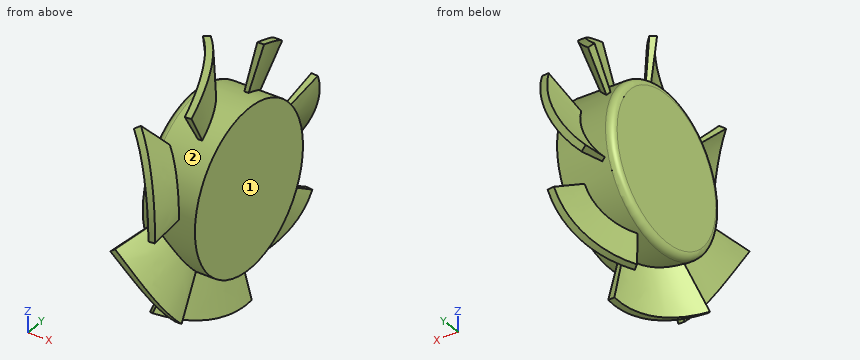
from build123d import *

# Parameters (mm, degrees)
SKETCH5_W                  = 8
SKETCH5_H                  = 11.5
CIRPATTERN1_COUNT          = 7
SKETCH_CUT_BLADE_OUTSIDE_W = 50.999
SKETCH_CUT_BLADE_OUTSIDE_H = 50.116
SKETCH_CUT_BLADE_OUTSIDE_R = 18
CUT_FAN_BLADE_DEPTH        = 30.009117079
COSMETIC_FILLET_R          = 1


with BuildPart() as part:
    # Sketch5 → Body (revolve)
    with BuildSketch(Plane.XY, mode=Mode.PRIVATE) as body_sk:
        with Locations((-6, 5.75)):
            Rectangle(SKETCH5_W, SKETCH5_H)
    revolve(body_sk.sketch.rotate(Axis((-10, 0, 0), (1, 0, 0)), 180), axis=Axis((-10, 0, 0), (1, 0, 0)))

    # Sketch-Blade-Top → Loft-Fan-Blade section 0
    with BuildSketch(Plane(origin=(0, 18, 0), x_dir=(-1, 0, 0), z_dir=(0, 1, 0)), mode=Mode.PRIVATE) as loft_fan_blade_s0:
        with BuildLine():
            Line((4.220534784, 7.137045162), (3.222970733, 7.067288688))
            ThreePointArc((3.222970733, 7.067288688), (5.086454542, -0.406736643), (9.393823742, -6.792674095))
            Line((9.393823742, -6.792674095), (10.113163542, -6.098015725))
            ThreePointArc((10.113163542, -6.098015725), (6, 0), (4.220534784, 7.137045162))
        make_face()
    loft_fan_blade = loft([loft_fan_blade_s0.sketch, Vertex(-6, 0, 0)])

    # CirPattern1: Loft-Fan-Blade ×7 about axis
    cirpattern1_axis = Axis((-10, 0, 0), (1, 0, 0))
    for i in range(1, CIRPATTERN1_COUNT):
        add(loft_fan_blade.rotate(cirpattern1_axis, i * 360 / CIRPATTERN1_COUNT))

    # Sketch-Cut-Blade outside → Cut-Fan-Blade (cut, through all)
    with BuildSketch(Plane(origin=(0, 0, 0), x_dir=(0, 0, -1), z_dir=(1, 0, 0))):
        with Locations((0.0385, -0.657)):
            Rectangle(SKETCH_CUT_BLADE_OUTSIDE_W, SKETCH_CUT_BLADE_OUTSIDE_H)
        Circle(SKETCH_CUT_BLADE_OUTSIDE_R, mode=Mode.SUBTRACT)
    extrude(amount=-CUT_FAN_BLADE_DEPTH, mode=Mode.SUBTRACT)

    # Cosmetic-Fillet
    cosmetic_fillet_edges = [part.edges().sort_by_distance(p)[0] for p in [
        (-10, 11.5, 0),
    ]]
    fillet(cosmetic_fillet_edges, radius=COSMETIC_FILLET_R)


solid = part.part
The listing builds one solid part. Answer for the finished solid, in the listing's coordinates (mm). Face numbers are marked on the shaded views. Give positions to 0.01 mm unless a question says otherwise; leave off trailing zeros. Use a Markdown table: item, result.
1. Find the intervals of material crossed by probe 1 along Y at (x, z) = (-4, -1.5); probe 2 along Z at (x, y) = (-6.25, 5); probe 3 along Y at (x, z) = (-8.5, 6.5), in increasing order. Write a range as from..to.
Values follow:
| item | result |
|---|---|
| probe 1 | y = -11.4..11.4 |
| probe 2 | z = -10.36..10.36 |
| probe 3 | y = -9.49..9.49, 9.97..10.35 |
2. For a pull along Z with two mould halves and no side action, classify the marked faces 1 and 2 as released by +Z, released by -Z, zero draft, split by the parting line, or undercut.
Values follow:
| item | result |
|---|---|
| face 1 | zero draft |
| face 2 | undercut |
3. Each of these flat-tipped pins is pushed along its axis until it touches: P1, Ø3, axis at x = -6.5, y = 1, coming from the +Z side; P2, Ø10, axis at y = -14, z = 13.5, coming from the -X side; P3, Ø2, axis at y = 12.5, z = 1, coming from the -X side; P4, Ø1.5, axis at x = -6, z = 8, coming from the -Y side. Where does it stop, or does it pass through?
Values follow:
| item | result |
|---|---|
| P1 | stops at z = 18 |
| P2 | stops at x = -9.9 |
| P3 | stops at x = -6 |
| P4 | stops at y = -16.46 |
